Verification items for the finished model (mm, model axes). Give positions to 0.01 mm unless a question says otherwise; leave off trailing zeros. Write each loop counter-clockwise with the first axis right and the second up, starting at its lowest first coordinate (ties: lowest second). Pieces come first, ordered by that corner, then holes.
from build123d import *

# Parameters (mm, degrees)
SKETCH1_W           = 203.2
SKETCH1_H           = 133.35
BOSS_EXTRUDE1_DEPTH = 3.175
SKETCH3_W           = 35.687
SKETCH3_H           = 3.175
BOSS_EXTRUDE2_DEPTH = 3.175
SKETCH4_W           = 3.175
SKETCH4_H           = 18.542
BOSS_EXTRUDE3_DEPTH = 3.175
SKETCH5_R           = 3.429
BOSS_EXTRUDE4_DEPTH = 3.175
SKETCH8_W           = 127
SKETCH8_H           = 76.2
CUT_EXTRUDE4_DEPTH  = 183.223979624


with BuildPart() as part:
    # Sketch1 → Boss-Extrude1 (new body)
    with BuildSketch(Plane(origin=(0, 0, 0), x_dir=(1, 0, 0), z_dir=(0, 1, 0))):
        Rectangle(SKETCH1_W, SKETCH1_H)
    extrude(amount=BOSS_EXTRUDE1_DEPTH)

    # Sketch3 → Boss-Extrude2 (add)
    with BuildSketch(Plane(origin=(0, 3.175, 0), x_dir=(1, 0, 0), z_dir=(0, 1, 0))):
        with Locations((-61.2775, 68.2625)):
            Rectangle(SKETCH3_W, SKETCH3_H)
        with Locations((0.3175, 68.2625)):
            Rectangle(SKETCH3_W, SKETCH3_H)
        with Locations((61.9125, 68.2625)):
            Rectangle(SKETCH3_W, SKETCH3_H)
        with Locations((61.9125, -68.2625)):
            Rectangle(SKETCH3_W, SKETCH3_H)
        with Locations((0.3175, -68.2625)):
            Rectangle(SKETCH3_W, SKETCH3_H)
        with Locations((-61.2775, -68.2625)):
            Rectangle(SKETCH3_W, SKETCH3_H)
    extrude(amount=-BOSS_EXTRUDE2_DEPTH)

    # Sketch4 → Boss-Extrude3 (add)
    with BuildSketch(Plane(origin=(0, 3.175, 0), x_dir=(1, 0, 0), z_dir=(0, 1, 0))):
        with Locations((-103.1875, 38.1)):
            Rectangle(SKETCH4_W, SKETCH4_H)
        with Locations((-103.1875, 0)):
            Rectangle(SKETCH4_W, SKETCH4_H)
        with Locations((-103.1875, -38.1)):
            Rectangle(SKETCH4_W, SKETCH4_H)
        with Locations((103.1875, -38.1)):
            Rectangle(SKETCH4_W, SKETCH4_H)
        with Locations((103.1875, 0)):
            Rectangle(SKETCH4_W, SKETCH4_H)
        with Locations((103.1875, 38.1)):
            Rectangle(SKETCH4_W, SKETCH4_H)
    extrude(amount=-BOSS_EXTRUDE3_DEPTH)

    # Sketch5 → Boss-Extrude4 (add)
    with BuildSketch(Plane(origin=(0, 3.175, 0), x_dir=(1, 0, 0), z_dir=(0, 1, 0))):
        Polygon((-104.775, 69.85), (-168.275, 69.85), (-168.275, -69.85), (-104.775, -69.85), (104.775, -69.85), (104.775, 69.85), align=None)
        with Locations(Location((-117.475, 57.15, 0), (0, 0, 270))):
            Circle(SKETCH5_R, mode=Mode.SUBTRACT)
        with Locations(Location((-130.175, 57.15, 0), (0, 0, 270))):
            Circle(SKETCH5_R, mode=Mode.SUBTRACT)
        with Locations(Location((-142.875, 57.15, 0), (0, 0, 270))):
            Circle(SKETCH5_R, mode=Mode.SUBTRACT)
        with Locations(Location((-155.575, 57.15, 0), (0, 0, 270))):
            Circle(SKETCH5_R, mode=Mode.SUBTRACT)
        with Locations(Location((-130.175, 44.45, 0), (0, 0, 270))):
            Circle(SKETCH5_R, mode=Mode.SUBTRACT)
        with Locations(Location((-142.875, 44.45, 0), (0, 0, 270))):
            Circle(SKETCH5_R, mode=Mode.SUBTRACT)
        with Locations(Location((-155.575, 44.45, 0), (0, 0, 270))):
            Circle(SKETCH5_R, mode=Mode.SUBTRACT)
        with Locations(Location((-130.175, 31.75, 0), (0, 0, 270))):
            Circle(SKETCH5_R, mode=Mode.SUBTRACT)
        with Locations(Location((-142.875, 31.75, 0), (0, 0, 270))):
            Circle(SKETCH5_R, mode=Mode.SUBTRACT)
        with Locations(Location((-155.575, 31.75, 0), (0, 0, 270))):
            Circle(SKETCH5_R, mode=Mode.SUBTRACT)
        with Locations(Location((-130.175, 19.05, 0), (0, 0, 270))):
            Circle(SKETCH5_R, mode=Mode.SUBTRACT)
        with Locations(Location((-142.875, 19.05, 0), (0, 0, 270))):
            Circle(SKETCH5_R, mode=Mode.SUBTRACT)
        with Locations(Location((-155.575, 19.05, 0), (0, 0, 270))):
            Circle(SKETCH5_R, mode=Mode.SUBTRACT)
        with Locations(Location((-130.175, 6.35, 0), (0, 0, 270))):
            Circle(SKETCH5_R, mode=Mode.SUBTRACT)
        with Locations(Location((-142.875, 6.35, 0), (0, 0, 270))):
            Circle(SKETCH5_R, mode=Mode.SUBTRACT)
        with Locations(Location((-155.575, 6.35, 0), (0, 0, 270))):
            Circle(SKETCH5_R, mode=Mode.SUBTRACT)
        with Locations(Location((-130.175, -6.35, 0), (0, 0, 270))):
            Circle(SKETCH5_R, mode=Mode.SUBTRACT)
        with Locations(Location((-142.875, -6.35, 0), (0, 0, 270))):
            Circle(SKETCH5_R, mode=Mode.SUBTRACT)
        with Locations(Location((-155.575, -6.35, 0), (0, 0, 270))):
            Circle(SKETCH5_R, mode=Mode.SUBTRACT)
        with Locations(Location((-130.175, -19.05, 0), (0, 0, 270))):
            Circle(SKETCH5_R, mode=Mode.SUBTRACT)
        with Locations(Location((-142.875, -19.05, 0), (0, 0, 270))):
            Circle(SKETCH5_R, mode=Mode.SUBTRACT)
        with Locations(Location((-155.575, -19.05, 0), (0, 0, 270))):
            Circle(SKETCH5_R, mode=Mode.SUBTRACT)
        with Locations(Location((-130.175, -31.75, 0), (0, 0, 270))):
            Circle(SKETCH5_R, mode=Mode.SUBTRACT)
        with Locations(Location((-142.875, -31.75, 0), (0, 0, 270))):
            Circle(SKETCH5_R, mode=Mode.SUBTRACT)
        with Locations(Location((-155.575, -31.75, 0), (0, 0, 270))):
            Circle(SKETCH5_R, mode=Mode.SUBTRACT)
        with Locations(Location((-130.175, -44.45, 0), (0, 0, 270))):
            Circle(SKETCH5_R, mode=Mode.SUBTRACT)
        with Locations(Location((-142.875, -44.45, 0), (0, 0, 270))):
            Circle(SKETCH5_R, mode=Mode.SUBTRACT)
        with Locations(Location((-155.575, -44.45, 0), (0, 0, 270))):
            Circle(SKETCH5_R, mode=Mode.SUBTRACT)
        with Locations(Location((-130.175, -57.15, 0), (0, 0, 270))):
            Circle(SKETCH5_R, mode=Mode.SUBTRACT)
        with Locations(Location((-142.875, -57.15, 0), (0, 0, 270))):
            Circle(SKETCH5_R, mode=Mode.SUBTRACT)
        with Locations(Location((-155.575, -57.15, 0), (0, 0, 270))):
            Circle(SKETCH5_R, mode=Mode.SUBTRACT)
        with Locations(Location((-117.475, 44.45, 0), (0, 0, 270))):
            Circle(SKETCH5_R, mode=Mode.SUBTRACT)
        with Locations(Location((-117.475, 31.75, 0), (0, 0, 270))):
            Circle(SKETCH5_R, mode=Mode.SUBTRACT)
        with Locations(Location((-117.475, 19.05, 0), (0, 0, 270))):
            Circle(SKETCH5_R, mode=Mode.SUBTRACT)
        with Locations(Location((-117.475, 6.35, 0), (0, 0, 270))):
            Circle(SKETCH5_R, mode=Mode.SUBTRACT)
        with Locations(Location((-117.475, -6.35, 0), (0, 0, 270))):
            Circle(SKETCH5_R, mode=Mode.SUBTRACT)
        with Locations(Location((-117.475, -19.05, 0), (0, 0, 270))):
            Circle(SKETCH5_R, mode=Mode.SUBTRACT)
        with Locations(Location((-117.475, -31.75, 0), (0, 0, 270))):
            Circle(SKETCH5_R, mode=Mode.SUBTRACT)
        with Locations(Location((-117.475, -44.45, 0), (0, 0, 270))):
            Circle(SKETCH5_R, mode=Mode.SUBTRACT)
        with Locations(Location((-117.475, -57.15, 0), (0, 0, 270))):
            Circle(SKETCH5_R, mode=Mode.SUBTRACT)
    extrude(amount=-BOSS_EXTRUDE4_DEPTH)

    # Sketch8 → Cut-Extrude4 (cut, through all)
    with BuildSketch(Plane(origin=(0, 0, 0), x_dir=(1, 0, 0), z_dir=(0, 1, 0))):
        with Locations((50.8, 0)):
            Rectangle(SKETCH8_W, SKETCH8_H)
    extrude(amount=CUT_EXTRUDE4_DEPTH, mode=Mode.SUBTRACT)


solid = part.part
Item 1: Sectioned sample at C-C on z = -44.45. Record the cut outline in (x, y) (3 decimals), then the cut area to 3 significant figures.
Answer key:
outline: (-168.275, 0) - (-159.004, 0) - (-159.004, 3.175) - (-168.275, 3.175) - close; (-152.146, 0) - (-146.304, 0) - (-146.304, 3.175) - (-152.146, 3.175) - close; (-139.446, 0) - (-133.604, 0) - (-133.604, 3.175) - (-139.446, 3.175) - close; (-126.746, 0) - (-120.904, 0) - (-120.904, 3.175) - (-126.746, 3.175) - close; (-114.046, 0) - (104.775, 0) - (104.775, 3.175) - (-114.046, 3.175) - close
area: 780 mm2
Item 2: Sectioned sample at D-D on y = 0.5. State how many separate pieces and enclosed holes the cut face has, then the cut area to 3 significant figures.
Answer key:
separate pieces: 1
enclosed holes: 40
area: 27,700 mm2
Item 3: Sectioned sample at B-B on z = 31.75. Record the cut outline in (x, y) (3 decimals), then the cut area to 3 significant figures.
Answer key:
outline: (-168.275, 0) - (-159.004, 0) - (-159.004, 3.175) - (-168.275, 3.175) - close; (-152.146, 0) - (-146.304, 0) - (-146.304, 3.175) - (-152.146, 3.175) - close; (-139.446, 0) - (-133.604, 0) - (-133.604, 3.175) - (-139.446, 3.175) - close; (-126.746, 0) - (-120.904, 0) - (-120.904, 3.175) - (-126.746, 3.175) - close; (-114.046, 0) - (-12.7, 0) - (-12.7, 3.175) - (-114.046, 3.175) - close
area: 407 mm2
Item 4: Depth check by flat-ended pin: pin 1 (5.5 mm diameter, centred on x = -142.875, z = 44.45, fed in from +Y); pin 2 (9 mm diameter, centred on x = -130.175, z = 31.75, fed in from -Y); pin 3 (1 mm diameter, centred on y = 0.5, z = 8.5, fed in from +X). Enter the tip coordinate at first touch or a pass-through.
Answer key:
pin 1: passes through
pin 2: stops at y = 0
pin 3: stops at x = -12.7
Item 5: Sectioned sample at A-A on x = 19. Record the cut outline in (y, z) (3 decimals).
Answer key:
outline: (0, -69.85) - (3.175, -69.85) - (3.175, -38.1) - (0, -38.1) - close; (0, 38.1) - (3.175, 38.1) - (3.175, 69.85) - (0, 69.85) - close
Item 6: Release check for a two-part mould opening along X. For faces 1 (the face through (-146.222, 1.61, 5.607)), 2 (the face through (-114.58, 1.61, 46.29)) record: released by +X, released by -X, zero draft, split by the parting line, or undercut.
Answer key:
face 1: undercut
face 2: undercut
Item 7: Scan lines: line 1 along X through (y, z) = (1.65, -44) (3 decimals); line 2 along Z through (x, y) = (68, 2.5); line 3 along X through (y, z) = (2.1, -6.35) (3 decimals). Record each from-to range of solid material in increasing order.
Answer key:
line 1: x = -168.275 to -158.974, -152.176 to -146.274, -139.476 to -133.574, -126.776 to -120.874, -114.076 to 104.775
line 2: z = -69.85 to -38.1, 38.1 to 69.85
line 3: x = -168.275 to -159.004, -152.146 to -146.304, -139.446 to -133.604, -126.746 to -120.904, -114.046 to -12.7
